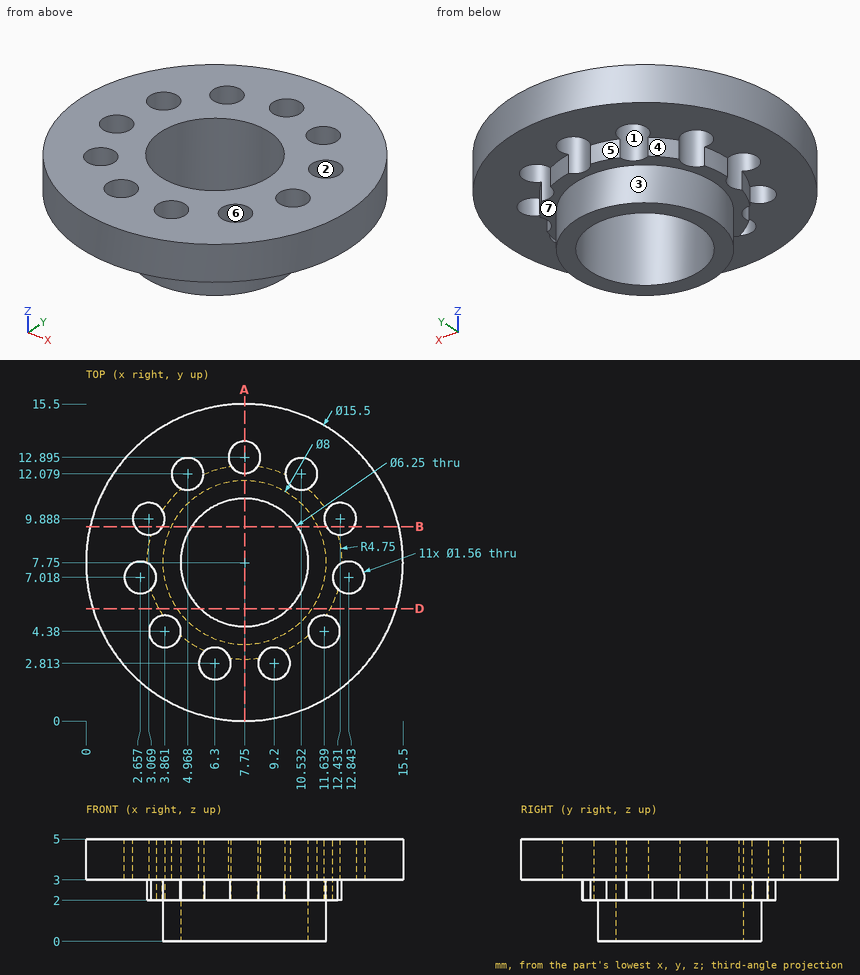
Verification items for this drawing (mm, ordinates from the low corner). A direction names the side the tool comes from. Round coordinates to 2 decimals unless told otherwise and drop trailing zeros. Loops run counter-clockwise (first coordinate to the right, second up) from the corner with the lowest first, then second, coordinate; pieces in that order, holes last. Notation, with made-up numbers: M 10.25,72.25 L 61.25,72.25 A30 cw 61.25,95.25 Z; hole C -21.75,-34 d4. An arc over 180 degrees is marked long. Answer as a JSON object with one key per item and string values.
1. Scan lines: line 1 (Y direction, x = 7.75, z = 3.5) (1 decimal); line 2 (Y direction, x = 7.75, z = 2.65) (1 decimal); line 3 (X direction, y = 2.25, z = 4.3). Record each from-to range of solid material in increasing order.
Reply:
{"line 1": "y = 0 to 4.6, 10.9 to 12.1, 13.7 to 15.5", "line 2": "y = 3 to 4.6, 10.9 to 12.1", "line 3": "x = 2.29 to 5.76, 6.84 to 8.66, 9.74 to 13.21"}
2. Section check B-B (y = 9.5). Record the boundary of the cut face in (x, z).
Reply:
{"outline": "M 0.2,3 L 2.39,3 L 2.39,5 L 0.2,5 Z; M 3.75,2 L 4.15,2 L 4.15,0 L 5.16,0 L 5.16,5 L 3.75,5 Z; M 10.34,0 L 11.35,0 L 11.35,2 L 11.75,2 L 11.75,5 L 10.34,5 Z; M 13.11,3 L 15.3,3 L 15.3,5 L 13.11,5 Z"}
3. Gauge pin test, flat ends, axial feed: P1, Ø1, axis at x = 13, z = 3, coming from the -Y side (1 decimal); P2, Ø1.2, axis at x = 4.97, y = 12.08, coming from the +Z side; P3, Ø1.8, axis at x = 12.43, y = 9.89, coming from the -Z side; P4, Ø1, axis at x = 13.5, z = 3, coming from the -Y side. Record the tip position at first contact, or that the pin passes through.
Reply:
{"P1": "stops at y = 1.6", "P2": "passes through", "P3": "stops at z = 2", "P4": "stops at y = 2.05"}
4. Access from +Z, -Z, +X, -X, +Y, -Y to the whole of each face (thin tool, end or side, straight path). Record for the marked faces 5, 6 and 7.
Reply:
{"face 5": "-Z, -X, +Y", "face 6": "+Z, -Z", "face 7": "-Z"}
5. Mould release check, pull along Y, two halves, no side actions. Record for the marked faces 1, 2, 3 and 4: pulls with the +Y half, pulls with the -Y half, needs draft (parallel to the pull), parting line crosses it, or undercut.
Reply:
{"face 1": "undercut", "face 2": "undercut", "face 3": "parting line crosses it", "face 4": "pulls with the +Y half"}
6. Section check D-D (y = 5.5). Record the boundary of the cut face in (x, z).
Reply:
{"outline": "M 0.33,3 L 3.57,3 L 3.57,2 L 4.44,2 L 4.44,0 L 5.58,0 L 5.58,5 L 0.33,5 Z; M 9.92,0 L 11.06,0 L 11.06,2 L 11.93,2 L 11.93,3 L 15.17,3 L 15.17,5 L 9.92,5 Z"}
7. Section check A-A (x = 7.75). State how many separate pieces and enclosed holes the cut face has.
Reply:
{"separate pieces": "3", "enclosed holes": "0"}
